The model under review builds one solid part; all positions refer to its coordinate system, in mm. Face numbers are marked on the shaded views. A direction names the side the tool comes from. Round coordinates to 2 decimals unless told otherwise and drop trailing zeros. Order: outer loops, then holes, each group sorted by start corner. A loop starts at its lowest first (then second) coordinate and runs counter-clockwise, first axis right, second up. Notation, with made-up numbers: M 69,20.5 L 81,20.5 A21 cw 81,51.5 Z; hole C 8,-26.5 d3. An arc over 180 degrees is marked long. Answer as a JSON object with one key per item and string values. Group by question number.
1. Add section A-A on y = 3. State the section outline as (x, z) points, and give its area (3 significant figures).
2. Machinability: for the marked faces 1, 2 and 3, which of the approach directions +Z, -Z, +X, -X, +Y, -Y give a long, thin tool a straight path to every point of the face, cutting with its end or side? Answer none if there is none.
3. Clearance check with a flat-ended pin moving along its axis: P1, Ø2.5, axis at x = 0, z = 5, coming from the +Y side. State where the tip first meets the part, or that it passes through.
4. Add section D-D on z = 1. State the section outline as (x, y) points, and give its area (3 significant figures).
5. To check wall thickness, follow probe 1 along X at (y, z) = (2.75, 2.25); probe 2 along Z at (x, y) = (0, 5.7); probe 3 along Y at (x, z) = (0, 8.25). State the ranges of each line that lie inside material, in increasing order. Write a range as [from, to].
6. Add section C-C on x = 0. State the section outline as (y, z) points.
7. Add section B-B on z = 5. State the section outline as (x, y) points.
8. Mouldability with a two-part tool opening along X and no side actions: class the marked faces 4, 5 and 6 as released by +X, released by -X, zero draft, split by the parting line, or undercut.
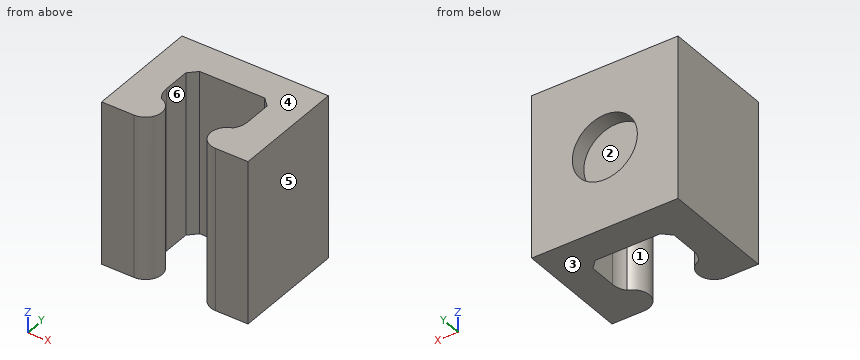
```python
from build123d import *

# Parameters (mm, degrees)
BOSS_EXTRUDE1_DEPTH = 10
SKETCH2_R           = 2
CUT_EXTRUDE1_DEPTH  = 1


with BuildPart() as part:
    # Sketch1 → Boss-Extrude1 (new body)
    with BuildSketch(Plane.XY):
        with BuildLine():
            Line((2.5, 1.798202453), (2.5, 3.5))
            Line((2.5, 3.5), (2, 4))
            Line((2, 4), (-2, 4))
            Line((-2, 4), (-2.5, 3.5))
            Line((-2.5, 3.5), (-2.5, 1.798202453))
            ThreePointArc((-2.5, 1.798202453), (-2.423157727, 1.350663613), (-2.2014329, 0.954388646))
            ThreePointArc((-2.2014329, 0.954388646), (-1.511468603, -0.151015487), (-2.5, -1))
            Line((-2.5, -1), (-4.5, -1))
            Line((-4.5, -1), (-4.5, 6))
            Line((-4.5, 6), (4.5, 6))
            Line((4.5, 6), (4.5, -1))
            Line((4.5, -1), (2.5, -1))
            ThreePointArc((2.5, -1), (1.511468603, -0.151015487), (2.2014329, 0.954388646))
            ThreePointArc((2.2014329, 0.954388646), (2.423157727, 1.350663613), (2.5, 1.798202453))
        make_face()
    extrude(amount=BOSS_EXTRUDE1_DEPTH)

    # Sketch2 → Cut-Extrude1 (cut)
    with BuildSketch(Plane(origin=(0, 6, 0), x_dir=(1, 0, 0), z_dir=(0, 1, 0))):
        with Locations(Location((0, -5, 0), (0, 0, 180))):
            Circle(SKETCH2_R)
    extrude(amount=-CUT_EXTRUDE1_DEPTH, mode=Mode.SUBTRACT)


solid = part.part
```
Recorded:
{
 "1": {"outline": "M -4.5,0 L -2.5,0 L -2.5,10 L -4.5,10 Z; M 2.5,0 L 4.5,0 L 4.5,10 L 2.5,10 Z", "area": "40.0 mm²"},
 "2": {"face 1": "+Z, -Z", "face 2": "+Y", "face 3": "-Z, +X, -X, +Y, -Y"},
 "3": {"P1": "stops at y = 5"},
 "4": {"outline": "M -4.5,-1 L -2.5,-1 A1 ccw -2.2,0.95 A1.34 cw -2.5,1.8 L -2.5,3.5 L -2,4 L 2,4 L 2.5,3.5 L 2.5,1.8 A1.34 cw 2.2,0.95 A1 ccw 2.5,-1 L 4.5,-1 L 4.5,6 L -4.5,6 Z", "area": "41.5 mm²"},
 "5": {"probe 1": "x = [-4.5, -2.5], [2.5, 4.5]", "probe 2": "z = [0, 3], [7, 10]", "probe 3": "y = [4, 6]"},
 "6": {"outline": "M 4,0 L 6,0 L 6,3 L 5,3 L 5,7 L 6,7 L 6,10 L 4,10 Z"},
 "7": {"outline": "M -4.5,-1 L -2.5,-1 A1 ccw -2.2,0.95 A1.34 cw -2.5,1.8 L -2.5,3.5 L -2,4 L 2,4 L 2.5,3.5 L 2.5,1.8 A1.34 cw 2.2,0.95 A1 ccw 2.5,-1 L 4.5,-1 L 4.5,6 L 2,6 L 2,5 L -2,5 L -2,6 L -4.5,6 Z"},
 "8": {"face 4": "zero draft", "face 5": "released by +X", "face 6": "undercut"}
}
